Job drawing, mm, ordinate dimensions from the low corner. One solid piece. Give positions to 0.01 mm unless a question says otherwise; leave off trailing zeros. Order: outer loops, then holes, each group sorted by start corner. A loop starts at its lowest first (then second) coordinate and runs counter-clockwise, first axis right, second up.
1. Drop flat-ended pins along their axis: pin 1 Ø3 at (x, y) = (15.88, 7.94) entering from +Z; pin 2 Ø3 at (y, z) = (11.5, 2) entering from -X; pin 3 Ø1.5 at (y, z) = (13, 5.5) entering from -X. Give the stop position or say it passes through.
2. Probe line 1 (X direction, y = 7, z = 0.5) (1 decimal); line 2 (X direction, y = 7.25, z = 6.25) (1 decimal); line 3 (Y direction, x = 94.5, z = 3.5). List the from-to ranges inside material, lowest first.
3. Slice it at A-A on z = 4.5. List the corners of the cut face in (x, y) (1 decimal), and give its area (3 significant figures).
4. Slice it at C-C on y = 14.5. List the corners of the cut face in (x, z), and give its area (3 significant figures).
5. Slice it at D-D on y = 3.5. List the corners of the cut face in (x, z), and give its area (3 significant figures).
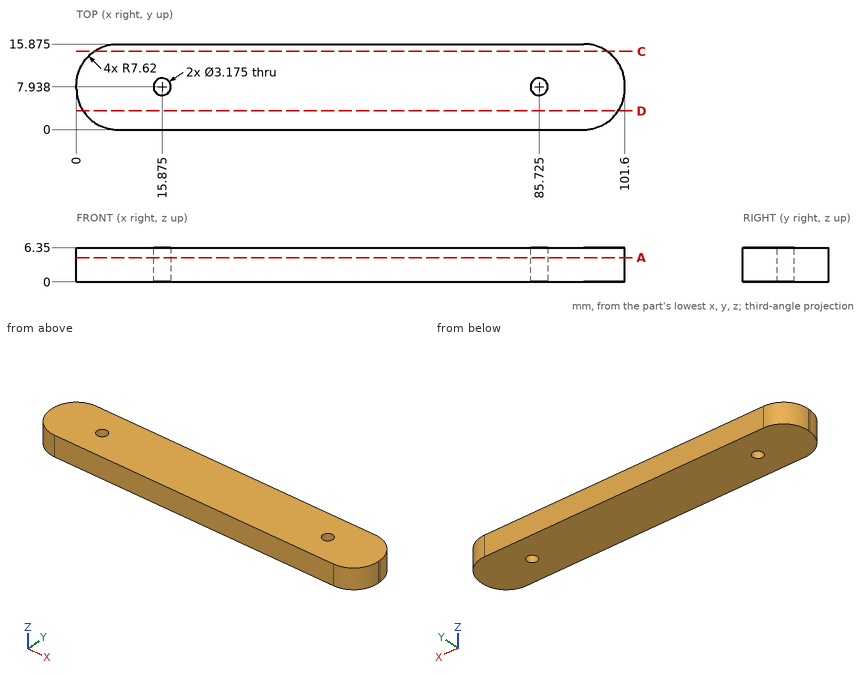
Data:
1. pin 1: passes through
1. pin 2: stops at x = 0.2
1. pin 3: stops at x = 1.13
2. line 1: x = 0 to 14.6, 17.2 to 84.4, 87 to 101.6
2. line 2: x = 0 to 14.4, 17.3 to 84.3, 87.2 to 101.6
2. line 3: y = 0.02 to 15.86
3. outline: (0, 7.6) arc R7.6 ccw to (7.6, 0) - (94, 0) arc R7.6 ccw to (101.6, 7.6) - (101.6, 8.3) arc R7.6 ccw to (94, 15.9) - (7.6, 15.9) arc R7.6 ccw to (0, 8.3) - close; hole circle Ø3.2 at (15.9, 7.9); hole circle Ø3.2 at (85.7, 7.9)
3. area: 1,550 mm2
4. outline: (3.25, 0) - (98.35, 0) - (98.35, 6.35) - (3.25, 6.35) - close
4. area: 604 mm2
5. outline: (1.21, 0) - (100.39, 0) - (100.39, 6.35) - (1.21, 6.35) - close
5. area: 630 mm2
